Can you work these out from the drawing? Everything is in mm from the part's minimum corner. A direction names the side the tool comes from. Coordinates: 2 decimals unless noted, no trailing zeros. Loops run counter-clockwise (first coordinate to the right, second up) from the corner with the lowest first, then second, coordinate; pieces in that order, holes last.
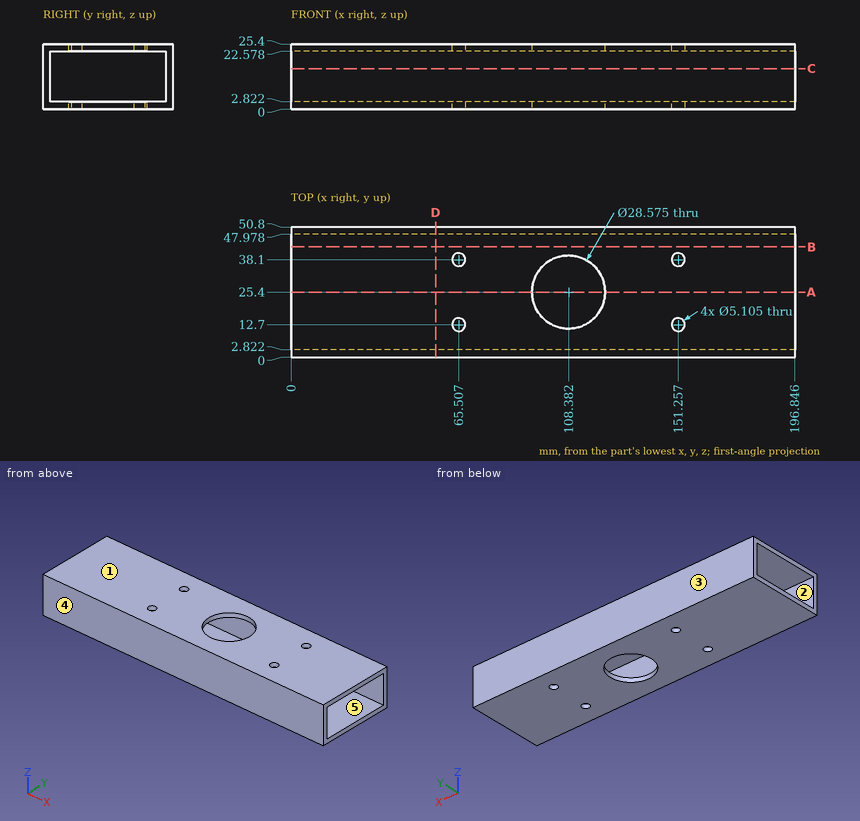
Item 1: We'd pull the mould along Y, two halves only. Please class the marked faces 3, 4 and 5: +Y half, -Y half, draft (parallel to the pull), parting line (faces both ways), or undercut.
Results are:
face 3: +Y half
face 4: -Y half
face 5: undercut
Item 2: I need wall thicknesses on line 1 along Z through (x, y) = (124.5, 38); line 2 along Y through (x, z) = (69.5, 3); line 3 along X through (y, z) = (25.4, 1.35) (1 decimal). Which ranges of each line are inside material? Lowest first, please.
Results are:
line 1: z = 0 to 2.82, 22.58 to 25.4
line 2: y = 0 to 2.82, 47.98 to 50.8
line 3: x = 0 to 94.1, 122.7 to 196.8
Item 3: On a 3-axis mill with a long thin cutter (end or side, diameter ignored), from which of +Z, -Z, +X, -X, +Y, -Y can I reach the whole of each face in a straight line? I mean the marked faces 1 and 2. Say none if no direction works.
Results are:
face 1: +Z, +X, -X, +Y, -Y
face 2: +X, -X
Item 4: I'm going to push a flat-ended pin straight in: P1, Ø3, axis at x = 65.51, y = 12.7, coming from the -Z side. Where does the tip first touch, or does it pass through?
Results are:
P1: passes through
Item 5: Suppose I cut it at C-C, the plane z = 15.75. Please give me the cut outline in (x, y).
Results are:
outline: (0, 0) - (196.85, 0) - (196.85, 2.82) - (0, 2.82) - close; (0, 47.98) - (196.85, 47.98) - (196.85, 50.8) - (0, 50.8) - close
Item 6: Suppose I cut it at D-D, the plane x = 56.5. Please give me the cut outline in (y, z), plus the area to 3 significant figures.
Results are:
outline: (0, 0) - (50.8, 0) - (50.8, 25.4) - (0, 25.4) - close; hole (2.82, 2.82) - (47.98, 2.82) - (47.98, 22.58) - (2.82, 22.58) - close
area: 398 mm2
Item 7: Suppose I cut it at A-A, the plane y = 25.4. Please give me the cut outline in (x, z) (1 decimal).
Results are:
outline: (0, 0) - (94.1, 0) - (94.1, 2.8) - (0, 2.8) - close; (0, 22.6) - (94.1, 22.6) - (94.1, 25.4) - (0, 25.4) - close; (122.7, 0) - (196.8, 0) - (196.8, 2.8) - (122.7, 2.8) - close; (122.7, 22.6) - (196.8, 22.6) - (196.8, 25.4) - (122.7, 25.4) - close
Item 8: Suppose I cut it at B-B, the plane y = 43. Please give me the cut outline in (x, z), plus the area to 3 significant figures.
Results are:
outline: (0, 0) - (196.85, 0) - (196.85, 2.82) - (0, 2.82) - close; (0, 22.58) - (196.85, 22.58) - (196.85, 25.4) - (0, 25.4) - close
area: 1,110 mm2
